The model under review builds one solid part; all positions refer to its coordinate system, in mm. Round coordinates to 2 decimals unless told otherwise and drop trailing zeros. Write each loop counter-clockwise with the first axis right and the second up, starting at its lowest first coordinate (ties: lowest second). Pieces come first, ordered by that corner, then holes. Notation, with made-up numbers: (-15, 85.5) - (15, 85.5) arc R32 ccw to (15, 120.5) - close; hole circle Ø9 at (-36, 79.25). An arc over 180 degrees is marked (long way). Return JSON: item names as keys, results as strings.
from build123d import *

# Parameters (mm, degrees)
SKETCH1_W           = 25.4
SKETCH1_H           = 30.48
BOSS_EXTRUDE1_DEPTH = 1.6
SKETCH2_R           = 1.09
CUT_EXTRUDE1_DEPTH  = 1.6


with BuildPart() as part:
    # Sketch1 → Boss-Extrude1 (new body)
    with BuildSketch(Plane(origin=(0, 0, 0), x_dir=(1, 0, 0), z_dir=(0, 1, 0))):
        Rectangle(SKETCH1_W, SKETCH1_H)
    extrude(amount=BOSS_EXTRUDE1_DEPTH)

    # Sketch2 → Cut-Extrude1 (cut)
    with BuildSketch(Plane(origin=(0, 1.6, 0), x_dir=(1, 0, 0), z_dir=(0, 1, 0))):
        with Locations(Location((-10.2, 12.74, 0), (0, 0, 270))):
            Circle(SKETCH2_R)
    cut_extrude1 = extrude(amount=-CUT_EXTRUDE1_DEPTH, mode=Mode.SUBTRACT)

    # Mirror1: Cut-Extrude1 across plane
    add(cut_extrude1.mirror(Plane.XY), mode=Mode.SUBTRACT)


solid = part.part
(1) Mouldability with a two-part tool opening along Z and no side actions: class faces 1 (the cylindrical face through (-11, 1, 12)), 2 (the flat face through (0, 1, -15.24)), 3 (the flat face through (0, 1.6, 0)) as released by +Z, released by -Z, zero draft, split by the parting line, or undercut.
Filled in:
{"face 1": "undercut", "face 2": "released by -Z", "face 3": "zero draft"}
(2) Add section B-B (x = -10.2). Write out the cut boundary in (y, z), plus the area to 3 significant figures.
Filled in:
{"outline": "(0, -15.24) - (1.6, -15.24) - (1.6, -13.83) - (0, -13.83) - close; (0, -11.65) - (1.6, -11.65) - (1.6, 11.65) - (0, 11.65) - close; (0, 13.83) - (1.6, 13.83) - (1.6, 15.24) - (0, 15.24) - close", "area": "41.8 mm2"}
(3) Wall thickness on line 1 (X direction, y = 1.05, z = 12.74); line 2 (Z direction, x = -9.75, y = 0.85): over which ranges is each line inside the solid? List them lowest first.
Filled in:
{"line 1": "x = -12.7 to -11.29, -9.11 to 12.7", "line 2": "z = -15.24 to -13.73, -11.75 to 11.75, 13.73 to 15.24"}
(4) Clearance check with a flat-ended pin moving along its axis: pin 1 Ø2 at (x, z) = (-2.5, -5) entering from -Y. State where the tip first meets the part, or that it passes through.
Filled in:
{"pin 1": "stops at y = 0"}
(5) Add section A-A (z = 12.74). Write out the cut boundary in (x, y), plus the area to 3 significant figures.
Filled in:
{"outline": "(-12.7, 0) - (-11.29, 0) - (-11.29, 1.6) - (-12.7, 1.6) - close; (-9.11, 0) - (12.7, 0) - (12.7, 1.6) - (-9.11, 1.6) - close", "area": "37.2 mm2"}
